from build123d import *

# Parameters (mm, degrees)
F0_W     = 101.8161997199
F0_H     = 45.5561242998
F1_DEPTH = 25.4
F1_TAPER = -3
F2_R     = 16.4012411608
F2_R_2   = 17.2999496767
F3_DEPTH = 29.4599
F4_R     = 5.08
F5_SIZE  = 5.08
F7_D     = 6.35


with BuildPart() as f1:
    # F0 (on Top) → F1 (new body)
    with BuildSketch(Plane.XY):
        with Locations((-50.90809986, 22.7780621499)):
            Rectangle(F0_W, F0_H)
    extrude(amount=F1_DEPTH, taper=F1_TAPER)

    # F2 (on face) → F3 (join)
    with BuildSketch(Plane.XY.offset(25.4)):
        with Locations((-66.870637238, 27.9236733913)):
            Circle(F2_R)
        with Locations((-21.7265021056, 26.3802520931)):
            Circle(F2_R_2)
    extrude(amount=F3_DEPTH)

    # F4
    f4_edges = [f1.edges().sort_by_distance(p)[0] for p in [
        (-102.481779, -0.665579, 12.7),
        (0.665579, -0.665579, 12.7),
        (0.665579, 46.221703, 12.7),
        (-102.481779, 46.221703, 12.7),
    ]]
    fillet(f4_edges, radius=F4_R)

    # F5
    f5_edges = [f1.edges().sort_by_distance(p)[0] for p in [
        (-39.026452, 26.380252, 54.8599),
        (-83.271878, 27.923673, 54.8599),
    ]]
    chamfer(f5_edges, length=F5_SIZE)

    # F7 (through all)
    with Locations(Plane.XY.offset(54.8599)):
        with Locations((-21.7265021056, 26.3802520931)):
            Hole(F7_D / 2)


solid = f1.part
Input: part model. Units: mm. Frame: model coordinates. A direction names the side the tool comes from. Give positions to 0.01 mm unless a question says otherwise; leave off trailing zeros. Answer as a JSON object with one key per item and string values. Group by question number.
Q1. Cut plane A-A, the plane z = 32. Count the separate pieces of the cut face and the enclosed holes in it, then the cut area to 3 significant figures.
Q2. Set-up query: faces 1 (the face through (-35.455, 15.854, 37.419)), 2 (the face through (-19, 24, 54.86)). Return all of +Z, -Z, +X, -X, +Y, -Y with unobstructed straight access to the full face (end or side cutting, diameter ignored); none if empty.
Q3. Mould query, pull axis Y, two halves, no side actions, for faces 3 (the face through (-83.256, 28.645, 37.419)), 4 (the face through (-21.04, 23.28, 27.05)), 5 (the face through (-52, 23, 0)). Classes: pulls with the +Y half, pulls with the -Y half, needs draft (parallel to the pull), parting line crosses it, or undercut.
Q4. First-contact query: pin 1 Ø5 at (y, z) = (27, 40.5) entering from -X; pin 2 Ø1 at (x, z) = (-41, 22) entering from +Y; pin 3 Ø10 at (y, z) = (32.5, 20) entering from -X; pin 4 Ø12 at (x, y) = (-48, 36.5) entering from -Z. Flat tips, straight axial feed; report the tip coordinate or a pass-through.
Q5. Line query: probe 1 along X at (y, z) = (25, 50); probe 2 along Z at (x, y) = (-28, 7.5); probe 3 along X at (y, z) = (38.5, 25.5) (3 decimals). Output: solid intervals per line, ascending.
Results:
{
 "1": {"separate pieces": "2", "enclosed holes": "1", "area": "1,750 mm^2"},
 "2": {"face 1": "+Z", "face 2": "+Z, +X, -X, +Y, -Y"},
 "3": {"face 3": "parting line crosses it", "face 4": "undercut", "face 5": "needs draft"},
 "4": {"pin 1": "x = -83.27", "pin 2": "y = 46.74", "pin 3": "x = -103.13", "pin 4": "z = 0"},
 "5": {"probe 1": "-82.79 to -50.96, -38.75 to -24.59, -18.87 to -4.7", "probe 2": "0 to 25.4", "probe 3": "-79.406 to -54.335, -34.072 to -9.381"}
}
